Source: CAD feature listing. Evaluate the final solid. Frame: model axes, mm. Face numbers are marked on the shaded views. A direction names the side the tool comes from. Give positions to 0.01 mm unless a question says otherwise; leave off trailing zeros. Loops run counter-clockwise (first coordinate to the right, second up) from the corner with the lowest first, then second, coordinate; pieces in that order, holes last. Notation, with made-up numbers: (52, -32.5) - (111, -32.5) arc R9 cw to (111, -28.5) - close; hole circle Ø4 at (4, 39.25). An arc over 180 degrees is marked (long way). Put each result on its own line as item: value.
```python
from build123d import *

# Parameters (mm, degrees)
F1_DEPTH  = 20
F3_D      = 12
F5_D      = 4.2
F5_DEPTH  = 14.4
F5_TIP    = 1.2618073
F6_SIZE   = 5
F7_W      = 60
F7_H      = 20
F8_DEPTH  = 30
F10_D     = 10.3
F11_W     = 29
F11_H     = 50
F12_DEPTH = 20.001


with BuildPart() as f1:
    # F0 (on Top) → F1 (new body)
    with BuildSketch(Plane.XY):
        Polygon((60, 0), (0, 0), (0, -55), (10, -55), (10, -20), (21, -20), (21, -55), (31, -55), (31, -20), (60, -20), align=None)
    extrude(amount=F1_DEPTH)

    # F3 (through all)
    with Locations(Plane(origin=(0, 0, 0), x_dir=(0, -1, 0), z_dir=(-1, 0, 0))):
        with Locations((43, 10)):
            Hole(F3_D / 2)

    # F5
    with Locations(Plane.XY.offset(20)):
        with Locations((5, -43), (26, -43)):
            Hole(F5_D / 2, depth=F5_DEPTH)
            with Locations((0, 0, -(F5_DEPTH + F5_TIP / 2))):  # 118° drill point
                Cone(0, F5_D / 2, F5_TIP, mode=Mode.SUBTRACT)

    # F6
    f6_edges = [f1.edges().sort_by_distance(p)[0] for p in [
        (5, -55, 20),
        (26, -55, 20),
        (26, -55, 0),
        (5, -55, 0),
    ]]
    chamfer(f6_edges, length=F6_SIZE)

    # F7 (on face) → F8 (join)
    with BuildSketch(Plane(origin=(0, 0, 0), x_dir=(-1, 0, 0), z_dir=(0, 1, 0))):
        with Locations((-30, 10)):
            Rectangle(F7_W, F7_H)
    extrude(amount=F8_DEPTH)

    # F10 (through all)
    with Locations(Plane.XY.offset(20)):
        with Locations((15.5, 17.5), (15.5, -7.5)):
            Hole(F10_D / 2)

    # F11 (on face) → F12 (cut, through all)
    with BuildSketch(Plane.XY.offset(20)):
        with Locations((45.5, 5)):
            Rectangle(F11_W, F11_H)
    extrude(amount=-F12_DEPTH, mode=Mode.SUBTRACT)


solid = f1.part
```
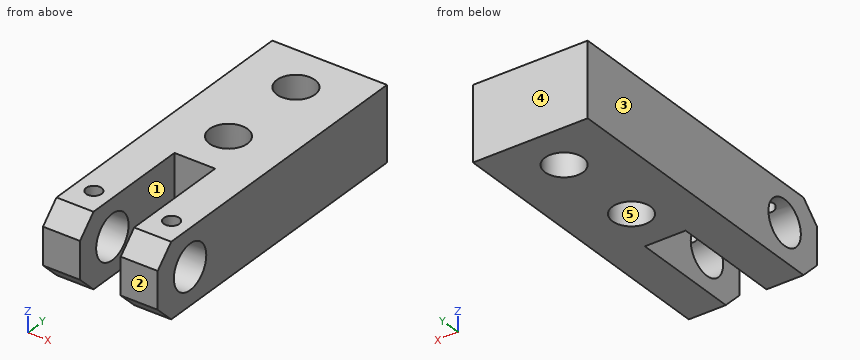
1) Section query C-C, the plane y = -34. Output: boundary loops of the cut face in (x, z), plus the area to 3 significant figures.
Check result:
outline: (0, 0) - (10, 0) - (10, 20) - (0, 20) - close; (21, 0) - (31, 0) - (31, 20) - (21, 20) - close
area: 400 mm²
2) Mould query, pull axis Y, two halves, no side actions, for the marked faces 3, 4 and 5. Classes: pulls with the +Y half, pulls with the -Y half, needs draft (parallel to the pull), parting line crosses it, or undercut.
Check result:
face 3: needs draft
face 4: pulls with the +Y half
face 5: undercut
3) Section query B-B, the plane x = 15.5. Output: boundary loops of the cut face in (y, z), plus the area to 3 significant figures.
Check result:
outline: (-20, 0) - (-12.65, 0) - (-12.65, 20) - (-20, 20) - close; (-2.35, 0) - (12.35, 0) - (12.35, 20) - (-2.35, 20) - close; (22.65, 0) - (30, 0) - (30, 20) - (22.65, 20) - close
area: 588 mm²
4) Access query for the marked faces 1 and 2. Directions: +Z, -Z, +X, -X, +Y, -Y. A direction counts if a zero-diameter tool reaches every point of the face in a straight line with its end or side. Return the directions, or none.
Check result:
face 1: +Z, -Z, -Y
face 2: +Z, -Z, +X, -X, -Y
5) Section query D-D, the plane z = 3. Output: boundary loops of the cut face in (x, y).
Check result:
outline: (0, -53) - (10, -53) - (10, -20) - (21, -20) - (21, -53) - (31, -53) - (31, 30) - (0, 30) - close; hole circle Ø10.3 at (15.5, -7.5); hole circle Ø10.3 at (15.5, 17.5)
6) Section query A-A, the plane z = 10. Output: boundary loops of the cut face in (x, y), plus the area to 3 significant figures.
Check result:
outline: (0, -55) - (10, -55) - (10, -49) - (0, -49) - close; (0, -37) - (10, -37) - (10, -20) - (21, -20) - (21, -37) - (31, -37) - (31, 30) - (0, 30) - close; (21, -55) - (31, -55) - (31, -49) - (21, -49) - close; hole circle Ø10.3 at (15.5, -7.5); hole circle Ø10.3 at (15.5, 17.5)
area: 1,840 mm²
7) Pin query (flat end, axial travel): P1, Ø1, axis at x = 14.5, y = -15.5, coming from the -Z side; P2, Ø11, axis at y = -43, z = 10, coming from the +X side. Return the tip coordinate at first contact, or that it passes through.
Check result:
P1: z = 0
P2: through
8) Material intervals for line 1 along X through (y, z) = (-43, 16.8); line 2 along X through (y, z) = (-31, 12.5); line 3 along Y through (x, z) = (12.5, 18.5), sorted ascending. Write a range as [from, to].
Check result:
line 1: [0, 2.9], [7.1, 10], [21, 23.9], [28.1, 31]
line 2: [0, 10], [21, 31]
line 3: [-20, -11.69], [-3.31, 13.31], [21.69, 30]
